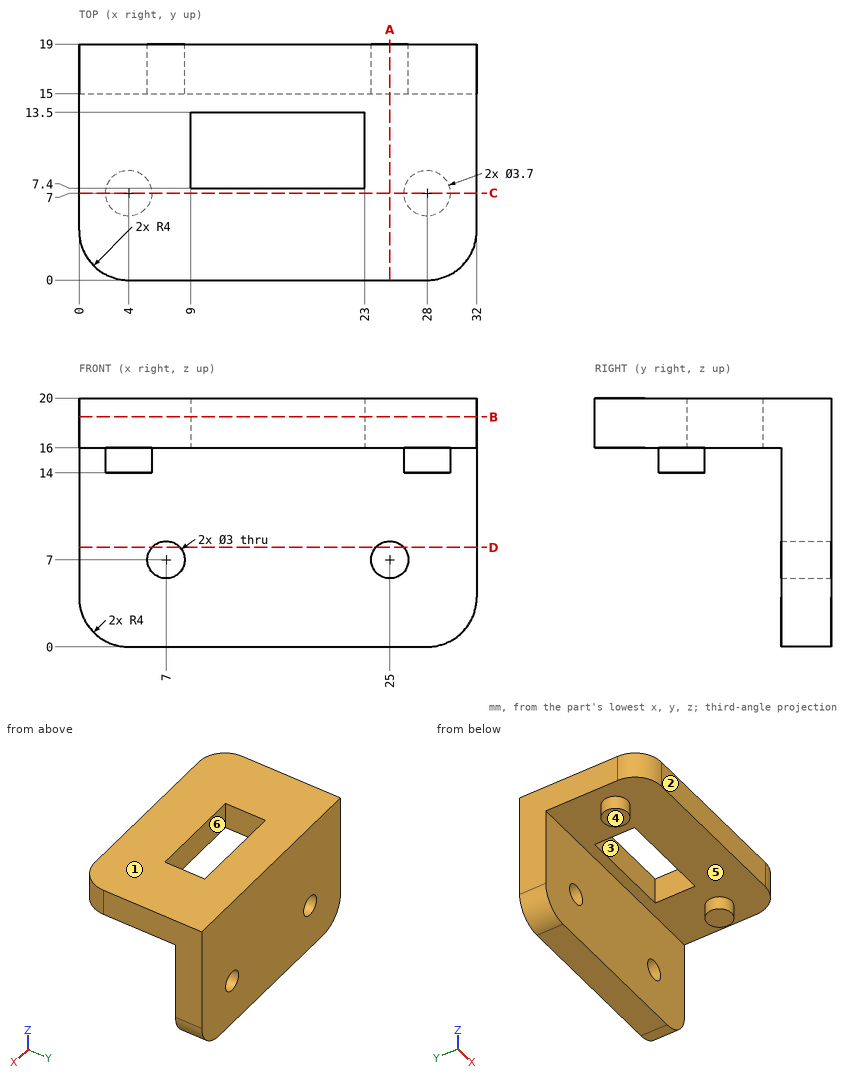
Source: three-view drawing plus pictorial views. Frame: mm from the lowest corner of the part. A direction names the side the tool comes from. Give positions to 0.01 mm unless a question says otherwise; leave off trailing zeros. Order: outer loops, then holes, each group sorted by start corner. A loop starts at its lowest first (then second) coordinate and runs counter-clockwise, first axis right, second up. Notation, with made-up numbers: M 8,24.5 L 28,24.5 A12 cw 28,40.5 Z; hole C 76,3.5 d4. An arc over 180 degrees is marked long. Return JSON: item names as keys, results as strings.
Item 1: Cut plane A-A (x = 25). Return loops of the section in (y, z).
Solutions:
{"outline": "M 0,16 L 15,16 L 15,8.5 L 19,8.5 L 19,20 L 0,20 Z; M 15,0 L 19,0 L 19,5.5 L 15,5.5 Z"}
Item 2: Ray query, probe 1 along Z at (x, y) = (6.5, 13); probe 2 along Z at (x, y) = (7, 16.5); probe 3 along Y at (x, z) = (27, 1). Return the intervals inside material, ascending.
Solutions:
{"probe 1": "16 to 20", "probe 2": "0 to 5.5, 8.5 to 20", "probe 3": "15 to 19"}
Item 3: First-contact query: P1, Ø3, axis at x = 9.5, z = 4.5, coming from the -Y side; P2, Ø7.5, axis at x = 17.5, y = 9.5, coming from the -Z side; P3, Ø3, axis at x = 28, y = 6.5, coming from the -Z side. Flat tips, straight axial feed; report the tip coordinate or a pass-through.
Solutions:
{"P1": "y = 15", "P2": "z = 16", "P3": "z = 14"}
Item 4: Access query for the marked faces 4, 5 and 6. Directions: +Z, -Z, +X, -X, +Y, -Y. A direction counts if a zero-diameter tool reaches every point of the face in a straight line with its end or side. Return the directions, or none.
Solutions:
{"face 4": "-Z, +X, -X, -Y", "face 5": "-Z", "face 6": "+Z, -Z"}
Item 5: Cut plane C-C (y = 7). Return loops of the section in (x, z), then the cut area to 3 significant figures.
Solutions:
{"outline": "M 0,16 L 2.15,16 L 2.15,14 L 5.85,14 L 5.85,16 L 26.15,16 L 26.15,14 L 29.85,14 L 29.85,16 L 32,16 L 32,20 L 0,20 Z", "area": "143 mm^2"}
Item 6: Cut plane B-B (z = 18.5). Return loops of the section in (x, y), then the cut area to 3 significant figures.
Solutions:
{"outline": "M 0,4 A4 ccw 4,0 L 28,0 A4 ccw 32,4 L 32,19 L 0,19 Z; hole M 9,7.4 L 23,7.4 L 23,13.5 L 9,13.5 Z", "area": "516 mm^2"}
Item 7: Pull-direction query (Y, two-part tool) for the marked faces 1, 2 and 3; classes: +Y half, -Y half, draft (parallel to the pull), parting line (faces both ways), or undercut.
Solutions:
{"face 1": "draft", "face 2": "-Y half", "face 3": "undercut"}
Item 8: Cut plane D-D (z = 8). Return loops of the section in (x, y).
Solutions:
{"outline": "M 0,15 L 5.88,15 L 5.88,19 L 0,19 Z; M 8.12,15 L 23.88,15 L 23.88,19 L 8.12,19 Z; M 26.12,15 L 32,15 L 32,19 L 26.12,19 Z"}
